```python
from build123d import *

# Parameters (mm, degrees)
BOSS_EXTRUDE1_DEPTH = 2.54
FILLET1_R           = 2.54
SKETCH2_W           = 27.305
SKETCH2_H           = 19.558
BOSS_EXTRUDE2_DEPTH = 2.413
SKETCH3_W           = 27.305
SKETCH3_H           = 14.605
BOSS_EXTRUDE3_DEPTH = 0.127


with BuildPart() as part:
    # Sketch1 → Boss-Extrude1 (new body)
    with BuildSketch(Plane(origin=(0, 0, 0), x_dir=(1, 0, 0), z_dir=(0, 1, 0))):
        Polygon((-6.163592518, 10.4775), (-9.2075, 13.6525), (-13.6525, 13.6525), (-13.6525, -13.6525), (13.6525, -13.6525), (13.6525, 13.6525), (9.2075, 13.6525), (5.895761697, 10.4775), align=None)
    extrude(amount=BOSS_EXTRUDE1_DEPTH)

    # Fillet1
    fillet1_edges = [part.edges().sort_by_distance(p)[0] for p in [
        (9.2075, 1.27, -13.6525),
        (13.6525, 1.27, -13.6525),
        (13.6525, 1.27, 13.6525),
        (-13.6525, 1.27, 13.6525),
        (-13.6525, 1.27, -13.6525),
        (-9.2075, 1.27, -13.6525),
        (-6.163592518, 1.27, -10.4775),
        (5.895761697, 1.27, -10.4775),
    ]]
    fillet(fillet1_edges, radius=FILLET1_R)

    # Sketch2 → Boss-Extrude2 (add)
    with BuildSketch(Plane(origin=(0, 2.54, 0), x_dir=(1, 0, 0), z_dir=(0, 1, 0))):
        with Locations((0, -0.8255)):
            Rectangle(SKETCH2_W, SKETCH2_H)
    extrude(amount=BOSS_EXTRUDE2_DEPTH)

    # Sketch3 → Boss-Extrude3 (add)
    with BuildSketch(Plane(origin=(0, 4.953, 0), x_dir=(1, 0, 0), z_dir=(0, 1, 0))):
        with Locations((0, -3.302)):
            Rectangle(SKETCH3_W, SKETCH3_H)
    extrude(amount=BOSS_EXTRUDE3_DEPTH)


solid = part.part
```
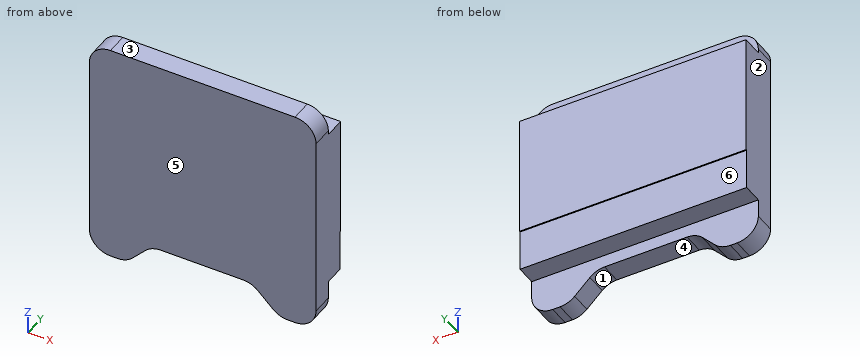
Input: part model. Units: mm. Frame: model coordinates. Face numbers are marked on the shaded views. A direction names the side the tool comes from. Give positions to 0.01 mm unless a question says otherwise; leave off trailing zeros. Write each loop counter-clockwise with the first axis right and the second up, starting at its lowest first coordinate (ties: lowest second). Pieces come first, ordered by that corner, then holes. Notation, with made-up numbers: (-26.5, 64.25) - (15.5, 64.25) arc R16 ccw to (15.5, 68.25) - close; hole circle Ø4 at (0, -19.75). An arc over 180 degrees is marked (long way). Write item = value, one per line. Start each with the question number.
1. Section query B-B, the plane x = -10.75. Output: boundary loops of the cut face in (y, z).
2. Section query D-D, the plane x = 12.25. Output: boundary loops of the cut face in (y, z).
3. Access query for the marked faces 4, 5 and 6. Directions: +Z, -Z, +X, -X, +Y, -Y. A direction counts if a zero-diameter tool reaches every point of the face in a straight line with its end or side. Return the directions, or none.
4. Ray query, L1, parallel to Z at x = -11.25, y = 3.3; L2, parallel to Y at x = 8.75, z = -8.75; L3, parallel to Z at x = 3.5, y = 2.1. Return the intervals inside material, ascending.
5. Mould query, pull axis X, two halves, no side actions, for the marked faces 1, 2 and 3. Classes: released by +X, released by -X, zero draft, split by the parting line, or undercut.
6. Section query C-C, the plane z = -6.25. Output: boundary loops of the cut face in (x, y).
7. Section query A-A, the plane y = 2.2. Output: boundary loops of the cut face in (x, z).
8. First-contact query: pin 1 Ø4 at (x, z) = (-1.5, -10.5) entering from +Y; pin 2 Ø2.5 at (x, y) = (-2.5, 3) entering from -Z; pin 3 Ø1.5 at (x, z) = (3.5, 12.5) entering from +Y. Flat tips, straight axial feed; report the tip coordinate or a pass-through.
Check sheet entries:
q1.outline = (0, -13.65) - (2.54, -13.65) - (2.54, -8.95) - (4.95, -8.95) - (4.95, -4) - (5.08, -4) - (5.08, 10.6) - (2.54, 10.6) - (2.54, 13.65) - (0, 13.65) - close
q2.outline = (0, -13.38) - (2.54, -13.38) - (2.54, -8.95) - (4.95, -8.95) - (4.95, -4) - (5.08, -4) - (5.08, 10.6) - (2.54, 10.6) - (2.54, 13.38) - (0, 13.38) - close
q3.face_4 = -Z, +Y, -Y
q3.face_5 = +Z, -Z, +X, -X, -Y
q3.face_6 = -Z, +X, -X, +Y
q4.L1 = -8.95 to 10.6
q4.L2 = 0 to 4.95
q4.L3 = -10.48 to 13.65
q5.face_1 = undercut
q5.face_2 = released by -X
q5.face_3 = zero draft
q6.outline = (-13.65, 0) - (13.65, 0) - (13.65, 4.95) - (-13.65, 4.95) - close
q7.outline = (-13.65, -11.11) arc R2.54 ccw to (-11.11, -13.65) - (-10.29, -13.65) arc R2.54 ccw to (-8.46, -12.87) - (-6.91, -11.26) arc R2.54 cw to (-5.08, -10.48) - (4.87, -10.48) arc R2.54 cw to (6.63, -11.18) - (8.47, -12.95) arc R2.54 ccw to (10.23, -13.65) - (11.11, -13.65) arc R2.54 ccw to (13.65, -11.11) - (13.65, 11.11) arc R2.54 ccw to (11.11, 13.65) - (-11.11, 13.65) arc R2.54 ccw to (-13.65, 11.11) - close
q8.pin_1 = 4.95
q8.pin_2 = -10.48
q8.pin_3 = 2.54
